from build123d import *

# Parameters (mm, degrees)
SKETCH1_W              = 50
SKETCH1_H              = 10.5
EXTRUDE_582_DEPTH      = 10
FILLET1_R              = 10
CUT_EXTRUDE_1185_REACH = 230.707
SKETCH2_R              = 1.5


with BuildPart() as part:
    # Sketch1 → Extrude 582 (new body)
    with BuildSketch(Plane.XY):
        Polygon((-225, 40), (-225, -40), (225, -30), (225, 30), align=None)
        with Locations((-80, -5)):
            Rectangle(SKETCH1_W, SKETCH1_H, mode=Mode.SUBTRACT)
        with Locations((120, -5)):
            Rectangle(SKETCH1_W, SKETCH1_H, mode=Mode.SUBTRACT)
    extrude(amount=EXTRUDE_582_DEPTH)

    # Fillet1
    fillet1_edges = [part.edges().sort_by_distance(p)[0] for p in [
        (225, 30, 5),
        (225, -30, 5),
        (-225, -40, 5),
        (-225, 40, 5),
    ]]
    fillet(fillet1_edges, radius=FILLET1_R)

    # Sketch2 → Cut-Extrude 1185 (cut, up to next)
    with BuildSketch(Plane.XY.offset(10), mode=Mode.PRIVATE) as cut_extrude_1185_sk1:
        with Locations((-165, -5)):
            Circle(SKETCH2_R)
    cut_extrude_1185_tool1 = extrude(cut_extrude_1185_sk1.sketch, amount=-CUT_EXTRUDE_1185_REACH, mode=Mode.PRIVATE) & part.part
    # Sketch2 → Cut-Extrude 1185 (cut, up to next)
    with BuildSketch(Plane.XY.offset(10), mode=Mode.PRIVATE) as cut_extrude_1185_sk2:
        with Locations((20, -5)):
            Circle(SKETCH2_R)
    cut_extrude_1185_tool2 = extrude(cut_extrude_1185_sk2.sketch, amount=-CUT_EXTRUDE_1185_REACH, mode=Mode.PRIVATE) & part.part
    # Sketch2 → Cut-Extrude 1185 (cut, up to next)
    with BuildSketch(Plane.XY.offset(10), mode=Mode.PRIVATE) as cut_extrude_1185_sk3:
        with Locations((185, -5)):
            Circle(SKETCH2_R)
    cut_extrude_1185_tool3 = extrude(cut_extrude_1185_sk3.sketch, amount=-CUT_EXTRUDE_1185_REACH, mode=Mode.PRIVATE) & part.part
    add(cut_extrude_1185_tool1.solids().sort_by_distance((-165, -5, 10))[0], mode=Mode.SUBTRACT)
    add(cut_extrude_1185_tool2.solids().sort_by_distance((20, -5, 10))[0], mode=Mode.SUBTRACT)
    add(cut_extrude_1185_tool3.solids().sort_by_distance((185, -5, 10))[0], mode=Mode.SUBTRACT)


solid = part.part
Work out the finished part from the listing and answer in its coordinate system (mm). A direction names the side the tool comes from. Coordinates: 2 decimals unless noted, no trailing zeros. Loops run counter-clockwise (first coordinate to the right, second up) from the corner with the lowest first, then second, coordinate; pieces in that order, holes last. Notation, with made-up numbers: (58, -24.75) -> (81, -24.75) arc R21 ccw to (81, 9.25) -> close; hole circle Ø4 at (63.25, 78.25). An arc over 180 degrees is marked (long way). Write each question's results on one line, items separated by ' | '. Start each with the question number.
1) Flat-ended cylindrical pins translate along their axes: P1, Ø2.5, axis at x = -165, y = -5, coming from the -Z side; P2, Ø3, axis at x = -73, z = 7, coming from the -Y side; P3, Ø6, axis at x = -96, z = 4.5, coming from the -Y side; P4, Ø6, axis at x = 152, z = 6.5, coming from the -Y side. Find the tip coordinate at first contact, or state that the pin passes through.
2) Find section B-B on z = 7.25. Determine the outline of the cut face in (x, y).
3) Consider line 1 along X through (y, z) = (-2.5, 3); line 2 along Y through (x, z) = (20, 6.5); line 3 along Y through (x, z) = (-165, 7.75). Determine where each line is inside the solid, lowest interval first.
4) Find section A-A on x = -63. Determine the outline of the cut face in (y, z).
5) For faces 1 (the flat face through (-80, -10.25, 5)), 2 (the cylindrical face through (222.07, 27.29, 5.07)), determine the directions among +Z, -Z, +X, -X, +Y, -Y from which every point of the face is accessible in a straight line to the end or side of a thin tool.
6) Find section C-C on x = -8. Determine the outline of the cut face in (y, z), then the cut area to 3 significant figures.
7) The mould has two halves that part along Y. Classify faces 3 (the flat face through (120, 0.25, 5)), 4 (the flat face through (120, -10.25, 5)), 5 (the flat face through (225, 0, 5)), 6 (the cylindrical face through (-222.07, 36.85, 5.07)): pulls with the +Y half, pulls with the -Y half, needs draft (parallel to the pull), parting line crosses it, or undercut.
Response values:
1) P1: passes through | P2: stops at y = -36.66 | P3: stops at y = -37.2 | P4: stops at y = -31.69
2) outline: (-225, -29.78) arc R10 ccw to (-214.78, -39.77) -> (215.22, -30.22) arc R10 ccw to (225, -20.22) -> (225, 20.22) arc R10 ccw to (215.22, 30.22) -> (-214.78, 39.77) arc R10 ccw to (-225, 29.78) -> close; hole circle Ø3 at (-165, -5); hole (-105, -10.25) -> (-55, -10.25) -> (-55, 0.25) -> (-105, 0.25) -> close; hole circle Ø3 at (20, -5); hole (95, -10.25) -> (145, -10.25) -> (145, 0.25) -> (95, 0.25) -> close; hole circle Ø3 at (185, -5)
3) line 1: x = -225 to -105, -55 to 95, 145 to 225 | line 2: y = -34.56 to -6.5, -3.5 to 34.56 | line 3: y = -38.67 to -6.5, -3.5 to 38.67
4) outline: (-36.4, 0) -> (-10.25, 0) -> (-10.25, 10) -> (-36.4, 10) -> close; (0.25, 0) -> (36.4, 0) -> (36.4, 10) -> (0.25, 10) -> close
5) face 1: +Z, -Z | face 2: +Z, -Z, +X, +Y
6) outline: (-35.18, 0) -> (35.18, 0) -> (35.18, 10) -> (-35.18, 10) -> close | area: 704 mm^2
7) face 3: undercut | face 4: undercut | face 5: needs draft | face 6: pulls with the +Y half
